Answer from the drawing. Dimensions are ordinates in mm from the lowest x, y and z of the part. Coordinates: 2 decimals unless noted, no trailing zeros. Write each loop counter-clockwise with the first axis right and the second up, starting at its lowest first coordinate (ties: lowest second). Pieces come first, ordered by that corner, then holes. Notation, with made-up numbers: (83.5, 1) -> (110.5, 1) arc R18 ccw to (110.5, 36) -> close; hole circle Ø10 at (44.5, 56). An arc over 180 degrees is marked (long way). One line per item, written item: value. Start each with the question number.
1. Find section C-C, the plane x = 21. Write down the section's boundary in (y, z).
2. Find section A-A, the plane z = 4.05. Write down the section's boundary in (x, y).
3. Find section D-D, the plane y = 5.75. Write down the section's boundary in (x, z).
4. For a pull along Y with two mould halves and no side action, classify the marked faces 1, 2 and 3 as pulls with the +Y half, pulls with the -Y half, needs draft (parallel to the pull), parting line crosses it, or undercut.
5. Find section B-B, the plane y = 2.5. Write down the section's boundary in (x, z).
6. Consider line 1 along X through (y, z) = (2.5, 2.15); line 2 along Y through (x, z) = (16.25, 3.7); line 3 along Y through (x, z) = (4, 2.4). Determine where each line is inside the solid, lowest interval first.
7. Given P1, Ø0.6, axis at x = 14.5, z = 3.5, coming from the +Y side; P2, Ø0.6, axis at x = 14.5, z = 3.5, coming from the -Y side; P3, Ø0.6, axis at x = 12, y = 3.5, coming from the +Z side, each flat-ended and moving along its own axis, determine where each tip first touches the part or whether it passes through.
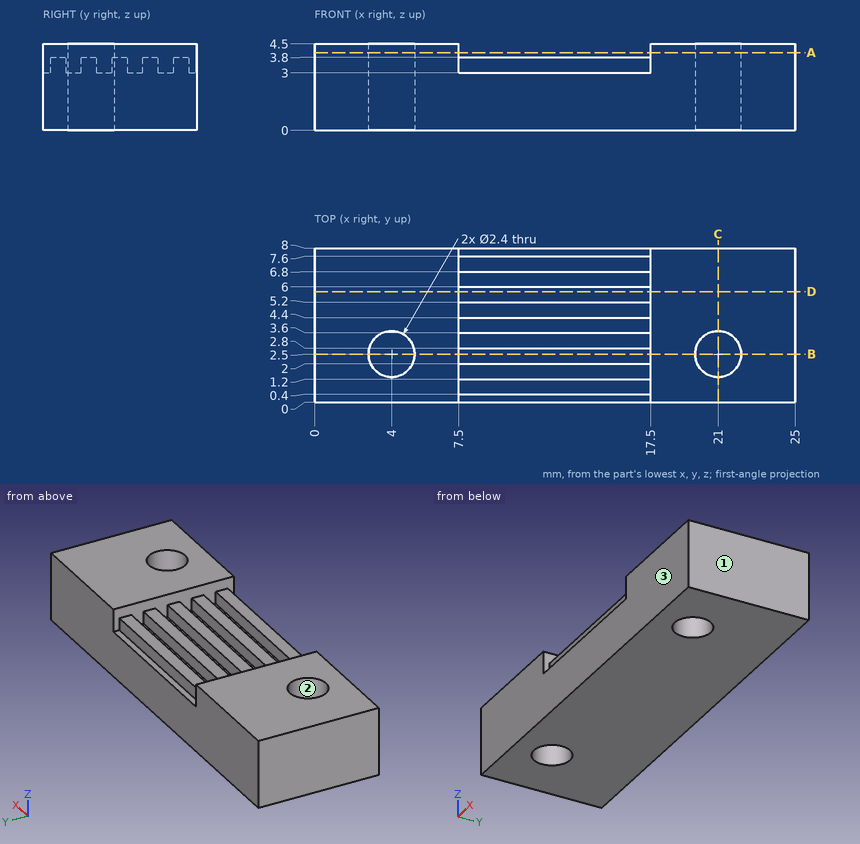
Answer block:
1. outline: (0, 0) -> (1.3, 0) -> (1.3, 4.5) -> (0, 4.5) -> close; (3.7, 0) -> (8, 0) -> (8, 4.5) -> (3.7, 4.5) -> close
2. outline: (0, 0) -> (7.5, 0) -> (7.5, 8) -> (0, 8) -> close; (17.5, 0) -> (25, 0) -> (25, 8) -> (17.5, 8) -> close; hole circle Ø2.4 at (4, 2.5); hole circle Ø2.4 at (21, 2.5)
3. outline: (0, 0) -> (25, 0) -> (25, 4.5) -> (17.5, 4.5) -> (17.5, 3.8) -> (7.5, 3.8) -> (7.5, 4.5) -> (0, 4.5) -> close
4. face 1: needs draft
4. face 2: undercut
4. face 3: pulls with the -Y half
5. outline: (0, 0) -> (2.8, 0) -> (2.8, 4.5) -> (0, 4.5) -> close; (5.2, 0) -> (19.8, 0) -> (19.8, 4.5) -> (17.5, 4.5) -> (17.5, 3.8) -> (7.5, 3.8) -> (7.5, 4.5) -> (5.2, 4.5) -> close; (22.2, 0) -> (25, 0) -> (25, 4.5) -> (22.2, 4.5) -> close
6. line 1: x = 0 to 2.8, 5.2 to 19.8, 22.2 to 25
6. line 2: y = 0.4 to 1.2, 2 to 2.8, 3.6 to 4.4, 5.2 to 6, 6.8 to 7.6
6. line 3: y = 0 to 1.3, 3.7 to 8
7. P1: stops at y = 7.6
7. P2: stops at y = 0.4
7. P3: stops at z = 3.8
